Design review of the part shown in the three views and the two pictorial views. Dimensions are in mm from the part's minimum x, y and z. Coordinates: 2 decimals unless noted, no trailing zeros. Order: outer loops, then holes, each group sorted by start corner. A loop starts at its lowest first (then second) coordinate and runs counter-clockwise, first axis right, second up. Notation, with made-up numbers: (26.5, 72) - (31.5, 72) arc R27 cw to (31.5, 96) - close; hole circle Ø10 at (89.25, -20). An arc over 180 degrees is marked (long way). One line per item, written item: value. Start each with the question number.
(1) Consider section D-D on y = 154. Write out the cut boundary in (x, z).
(2) To check wall thickness, follow line 1 along Y through (x, z) = (419, 3); line 2 along X through (y, z) = (175, 1); line 3 along Y through (x, z) = (105.5, 6.5). State the ranges of each line that lie inside material, in increasing order.
(3) Consider section A-A on x = 188. Write out the cut boundary in (y, z).
(4) Consider section C-C on x = 48.5. Write out the cut boundary in (y, z).
(5) Clearance check with flat-ended pins moving along their axes: pin 1 (5 mm diameter, centred on x = 425.5, z = 5.5, fed in from -Y); pin 2 (5 mm diameter, centred on y = 268.5, z = 5.5, fed in from -X); pin 3 (6 mm diameter, centred on y = 87, z = 5, fed in from -X); pin 4 (2 mm diameter, centred on y = 136.5, z = 8, fed in from -X). State where each tip first meets the part, or that it passes through.
(6) Consider section B-B on z = 1.75. Write out the cut boundary in (x, y), then the cut area to 3 significant figures.
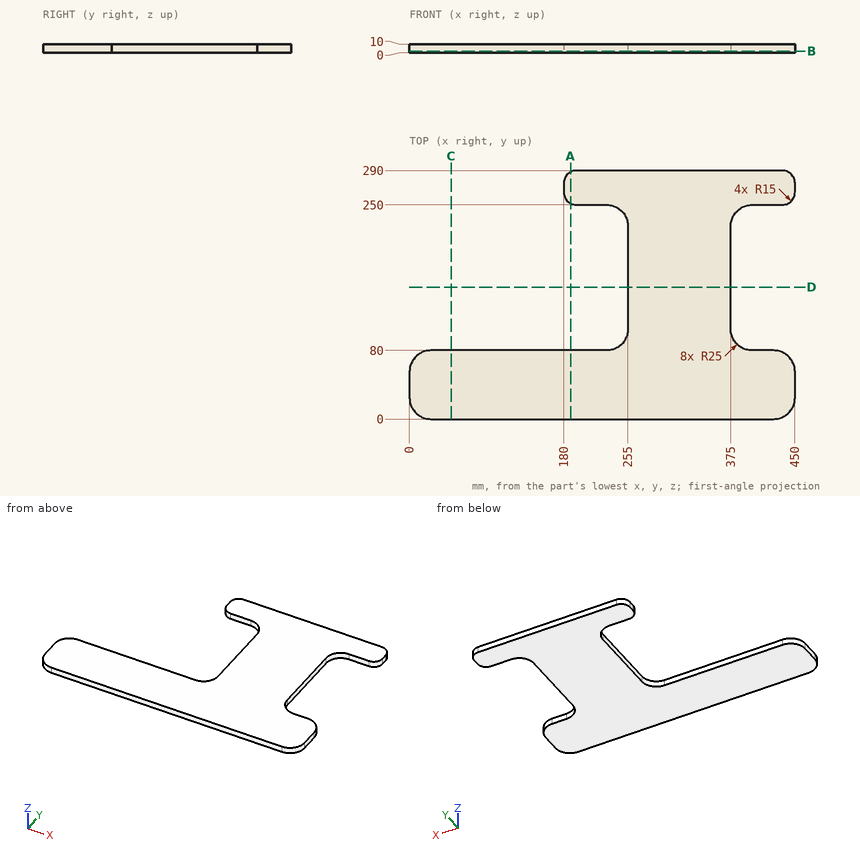
Geometry check:
1. outline: (255, 0) - (375, 0) - (375, 10) - (255, 10) - close
2. line 1: y = 0 to 80, 250 to 290
2. line 2: x = 255 to 375
2. line 3: y = 0 to 80
3. outline: (0, 0) - (80, 0) - (80, 10) - (0, 10) - close; (251.73, 0) - (288.27, 0) - (288.27, 10) - (251.73, 10) - close
4. outline: (0, 0) - (80, 0) - (80, 10) - (0, 10) - close
5. pin 1: stops at y = 0
5. pin 2: stops at x = 180
5. pin 3: stops at x = 243.56
5. pin 4: stops at x = 255
6. outline: (0, 25) arc R25 ccw to (25, 0) - (425, 0) arc R25 ccw to (450, 25) - (450, 55) arc R25 ccw to (425, 80) - (400, 80) arc R25 cw to (375, 105) - (375, 225) arc R25 cw to (400, 250) - (435, 250) arc R15 ccw to (450, 265) - (450, 275) arc R15 ccw to (435, 290) - (195, 290) arc R15 ccw to (180, 275) - (180, 265) arc R15 ccw to (195, 250) - (230, 250) arc R25 cw to (255, 225) - (255, 105) arc R25 cw to (230, 80) - (25, 80) arc R25 ccw to (0, 55) - close
6. area: 67,000 mm^2
